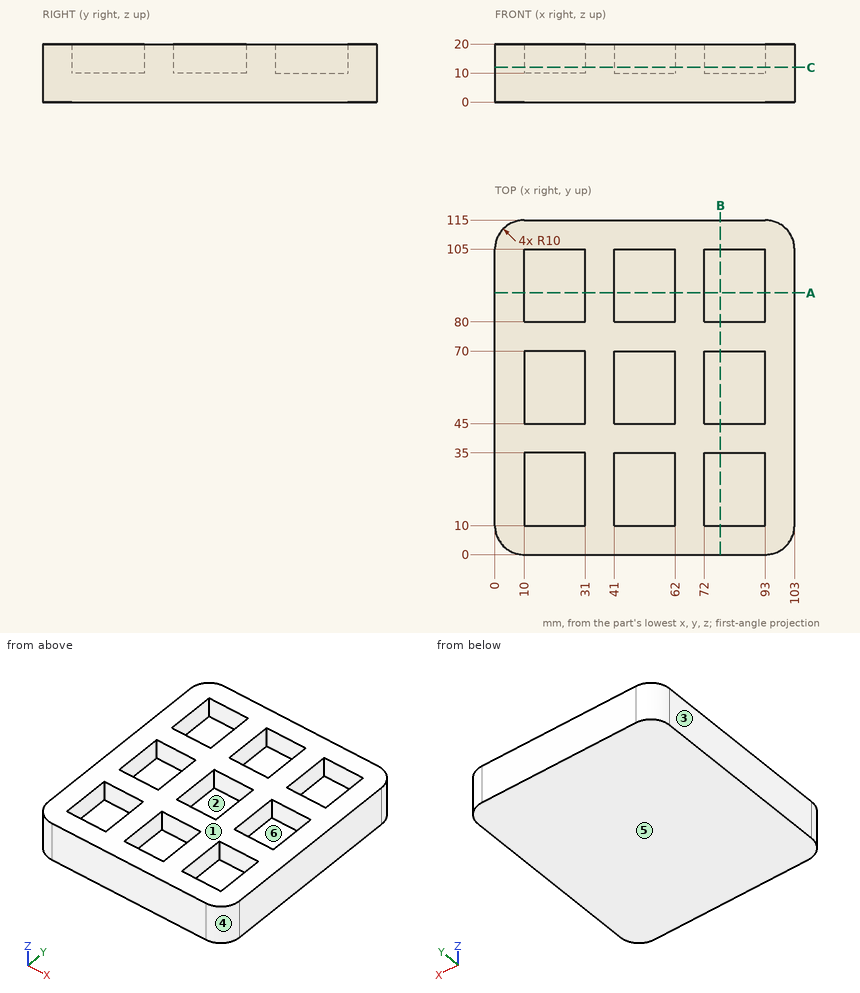
Geometry check sheet. Reference: drawing and pictorial views, mm from the part's lowest x, y, z. A direction names the side the tool comes from. Give positions to 0.01 mm unless a question says otherwise; leave off trailing zeros. Order: outer loops, then holes, each group sorted by start corner. A loop starts at its lowest first (then second) coordinate and runs counter-clockwise, first axis right, second up. Notation, with made-up numbers: M 86.5,17 L 117.5,17 A8 ccw 117.5,28 Z; hole C -32,10 d9. An arc over 180 degrees is marked long. Use one line per item in the form item = value. Start each with the question number.
Q1. Mould release check, pull along X, two halves, no side actions. Record for the marked faces 1, 2, 3 and 4: +X half, -X half, draft (parallel to the pull), parting line (faces both ways), or undercut.
Q2. Go/stop test with a flat-tipped pin: pin 1 Ø10.5 at (x, y) = (87.5, 93) entering from +Z. Record where the tip stops, or that it passes through.
Q3. Section check C-C (z = 12). Count the separate pieces of the cut face and the enclosed holes in it, then the cut area to 3 significant figures.
Q4. Access from +Z, -Z, +X, -X, +Y, -Y to the whole of each face (thin tool, end or side, straight path). Record for the marked faces 5 and 6.
Q5. Section check A-A (y = 90). Enter the section's corners in (x, z), then the cut area to 3 significant figures.
Q6. Scan lines: line 1 along Y through (x, z) = (12, 19.25); line 2 along X through (y, z) = (66, 11.25); line 3 along Z through (x, y) = (53, 54). Record each from-to range of solid material in increasing order. Write a range as [from, to].
Q7. Section check B-B (x = 77.5). Enter the section's corners in (y, z).
Evaluation:
q1.face_1 = draft
q1.face_2 = undercut
q1.face_3 = -X half
q1.face_4 = +X half
q2.pin_1 = 10
q3.separate_pieces = 1
q3.enclosed_holes = 9
q3.area = 7,030 mm2
q4.face_5 = -Z, +X, -X, +Y, -Y
q4.face_6 = +Z
q5.outline = M 0,0 L 103,0 L 103,20 L 93,20 L 93,10 L 72,10 L 72,20 L 62,20 L 62,10 L 41,10 L 41,20 L 31,20 L 31,10 L 10,10 L 10,20 L 0,20 Z
q5.area = 1,430 mm2
q6.line_1 = [0, 10], [35, 45], [70, 80], [105, 115]
q6.line_2 = [0, 10], [31, 41], [62, 72], [93, 103]
q6.line_3 = [0, 10]
q7.outline = M 0,0 L 115,0 L 115,20 L 105,20 L 105,10 L 80,10 L 80,20 L 70,20 L 70,10 L 45,10 L 45,20 L 35,20 L 35,10 L 10,10 L 10,20 L 0,20 Z
